Can you work these out from the model? Positions are in its coordinate system, mm. Face numbers are marked on the shaded views. A direction names the side the tool comes from. Give positions to 0.01 mm unless a question says otherwise; leave off trailing zeros. Order: outer loops, then holes, each group sorted by start corner. A loop starts at its lowest first (then second) coordinate and runs counter-clockwise, first axis right, second up. Notation, with made-up numbers: (42.5, -1) - (49.5, -1) arc R23 ccw to (49.5, 19) - close; hole circle Ø11 at (88, -18). An arc over 180 degrees is marked (long way). Answer as a JSON object with one key per item and string values.
```python
from build123d import *

# Parameters (mm, degrees)
SKETCH_1_W          = 54
SKETCH_1_H          = 91
SKETCH_1_W_2        = 50
SKETCH_1_H_2        = 87
EXTRUDE_1_DEPTH     = 17
SKETCH_2_W          = 54
SKETCH_2_H          = 91
EXTRUDE_2_DEPTH     = 2
SKETCH_3_W          = 12
SKETCH_3_H          = 98.630911944
CUT_EXTRUDE_1_DEPTH = 15
SKETCH_5_R          = 0.85
CUT_EXTRUDE_2_DEPTH = 11
FILLET_1_SIZE       = 1
FILLET_2_SIZE       = 5


with BuildPart() as part:
    # 草图1 → 凸台-拉伸1 (new body)
    with BuildSketch(Plane.XY):
        Rectangle(SKETCH_1_W, SKETCH_1_H)
        Rectangle(SKETCH_1_W_2, SKETCH_1_H_2, mode=Mode.SUBTRACT)
    extrude(amount=EXTRUDE_1_DEPTH)

    # 草图2 → 凸台-拉伸2 (add)
    with BuildSketch(Plane(origin=(0, 0, 0), x_dir=(-1, 0, 0), z_dir=(0, 0, -1))):
        Rectangle(SKETCH_2_W, SKETCH_2_H)
    extrude(amount=-EXTRUDE_2_DEPTH)

    # 草图3 → 切除-拉伸1 (cut)
    with BuildSketch(Plane.XY.offset(17)):
        Rectangle(SKETCH_3_W, SKETCH_3_H)
    extrude(amount=-CUT_EXTRUDE_1_DEPTH, mode=Mode.SUBTRACT)

    # 草图5 → 切除-拉伸2 (cut)
    with BuildSketch(Plane(origin=(0, 45.5, 0), x_dir=(1, 0, 0), z_dir=(0, 1, 0))):
        with Locations(Location((-9, -4.4, 0), (0, 0, 270))):
            Circle(SKETCH_5_R)
        with Locations(Location((-13, -7.6, 0), (0, 0, 270))):
            Circle(SKETCH_5_R)
        with Locations(Location((9, -4.4, 0), (0, 0, 270))):
            Circle(SKETCH_5_R)
        with Locations(Location((13, -7.6, 0), (0, 0, 270))):
            Circle(SKETCH_5_R)
    extrude(amount=-CUT_EXTRUDE_2_DEPTH, mode=Mode.SUBTRACT)

    # 圆角1
    # a fillet whose section is not a circle: 1 mm, written as the material it takes off along each edge
    with BuildSketch(Plane(origin=(-27, -45.5, -2.5), x_dir=(0, 1, 0), z_dir=(0, 0, 1)), Plane(origin=(27, -45.5, 19.5), x_dir=(0, 1, 0), z_dir=(0, 0, -1)), Plane(origin=(27, 45.5, 19.5), x_dir=(-1, 0, 0), z_dir=(0, 0, -1)), Plane(origin=(-27, 45.5, -2.5), x_dir=(1, 0, 0), z_dir=(0, 0, 1))) as fillet_1_piece_1:
        with BuildLine():
            add(Edge.make_bspline([(FILLET_1_SIZE, 0), (FILLET_1_SIZE * 0.831801948466, 0), (FILLET_1_SIZE * 0.663603896932, 0), (FILLET_1_SIZE * 0.292893218813, -FILLET_1_SIZE * 0.0716919198361), (FILLET_1_SIZE * 0.0716919198361, -FILLET_1_SIZE * 0.292893218813), (0, -FILLET_1_SIZE * 0.663603896932), (0, -FILLET_1_SIZE * 0.831801948466), (0, -FILLET_1_SIZE)], knots=[0, 0, 0, 0, 0, 0, 0.5, 0.5, 1, 1, 1, 1, 1, 1], degree=5))
            Line((0, -FILLET_1_SIZE), (0, 0))
            Line((0, 0), (FILLET_1_SIZE, 0))
        make_face()
    extrude(amount=22, mode=Mode.SUBTRACT)

    # 圆角2
    # a fillet whose section is not a circle: 5 mm, written as the material it takes off along each edge
    with BuildSketch(Plane(origin=(6, -31, 17), x_dir=(1, 0, 0), z_dir=(0, -1, 0)), Plane(origin=(-6, -58, 17), x_dir=(-1, 0, 0), z_dir=(0, 1, 0)), Plane(origin=(6, 58, 17), x_dir=(1, 0, 0), z_dir=(0, -1, 0))) as fillet_2_piece_1:
        with BuildLine():
            add(Edge.make_bspline([(FILLET_2_SIZE, 0), (FILLET_2_SIZE * 0.831801948466, 0), (FILLET_2_SIZE * 0.663603896932, 0), (FILLET_2_SIZE * 0.292893218813, -FILLET_2_SIZE * 0.0716919198361), (FILLET_2_SIZE * 0.0716919198361, -FILLET_2_SIZE * 0.292893218813), (0, -FILLET_2_SIZE * 0.663603896932), (0, -FILLET_2_SIZE * 0.831801948466), (0, -FILLET_2_SIZE)], knots=[0, 0, 0, 0, 0, 0, 0.5, 0.5, 1, 1, 1, 1, 1, 1], degree=5))
            Line((0, -FILLET_2_SIZE), (0, 0))
            Line((0, 0), (FILLET_2_SIZE, 0))
        make_face()
    extrude(amount=27, mode=Mode.SUBTRACT)
    with BuildSketch(Plane(origin=(-6, 31, 17), x_dir=(0, 0, -1), z_dir=(0, 1, 0))) as fillet_2_piece_2:
        with BuildLine():
            add(Edge.make_bspline([(FILLET_2_SIZE, 0), (FILLET_2_SIZE * 0.831801948466, 0), (FILLET_2_SIZE * 0.663603896932, 0), (FILLET_2_SIZE * 0.292893218813, FILLET_2_SIZE * 0.0716919198361), (FILLET_2_SIZE * 0.0716919198361, FILLET_2_SIZE * 0.292893218813), (0, FILLET_2_SIZE * 0.663603896932), (0, FILLET_2_SIZE * 0.831801948466), (0, FILLET_2_SIZE)], knots=[0, 0, 0, 0, 0, 0, 0.5, 0.5, 1, 1, 1, 1, 1, 1], degree=5))
            Line((0, FILLET_2_SIZE), (0, 0))
            Line((0, 0), (FILLET_2_SIZE, 0))
        make_face()
    extrude(amount=27, mode=Mode.SUBTRACT)


solid = part.part
```
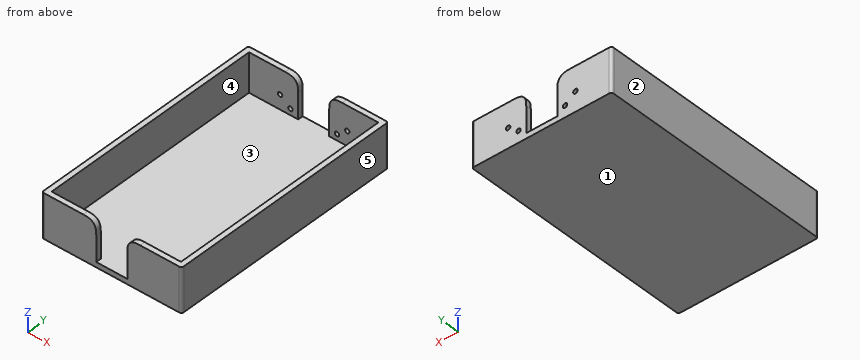
Q1. I'm going to push flat-ended pins straight in: pin 1 Ø15 at (x, y) = (0, 13) entering from +Z; pin 2 Ø1.4 at (x, z) = (-9, 4.4) entering from +Y. Where does each tip first touch, or does it pass through?
Recorded:
{"pin 1": "stops at z = 2", "pin 2": "stops at y = -43.5"}
Q2. We'd pull the mould along X, two halves only. Please class the marked faces 1, 2 and 3: released by +X, released by -X, zero draft, split by the parting line, or undercut.
Recorded:
{"face 1": "zero draft", "face 2": "released by -X", "face 3": "undercut"}
Q3. If we section it at B-B, the plane y = 9.5: Please give me the cut outline in (x, z), then the cut area to 3 significant figures.
Recorded:
{"outline": "(-27, 0) - (27, 0) - (27, 17) - (25, 17) - (25, 2) - (-25, 2) - (-25, 17) - (-27, 17) - close", "area": "168 mm^2"}
Q4. I need wall thicknesses on L1, parallel to X at y = 43.95, z = 7.6; L2, parallel to X at y = 35.5, z = 7.25; L3, parallel to Y at x = 24.5, z = 12.25. Which ranges of each line are inside material? Lowest first, please.
Recorded:
{"L1": "x = -27 to -13.85, -12.15 to -6, 6 to 12.15, 13.85 to 27", "L2": "x = -27 to -25, 25 to 27", "L3": "y = -45.5 to -43.5, 43.5 to 45.5"}
Q5. If we section it at C-C, the plane x = -1: Please give me the cut outline in (y, z).
Recorded:
{"outline": "(-45.5, 0) - (45.5, 0) - (45.5, 2) - (-45.5, 2) - close"}
Q6. Which directions (+Z, -Z, +X, -X, +Y, -Y) give clear straight access to the entire face, cutting with the end or side of a thin tool? Please do the marked faces 4 and 5.
Recorded:
{"face 4": "+Z", "face 5": "+Z, -Z, +X, +Y, -Y"}
Q7. If we section it at A-A, the plane x = -21.5: Please give me the cut outline in (y, z), then the cut area to 3 significant figures.
Recorded:
{"outline": "(-45.5, 0) - (45.5, 0) - (45.5, 17) - (43.5, 17) - (43.5, 2) - (-43.5, 2) - (-43.5, 17) - (-45.5, 17) - close", "area": "242 mm^2"}
